Here's the drawing with two shaded views (mm, measured from the low corner). I have some questions. A direction names the side the tool comes from. Round coordinates to 2 decimals unless told otherwise and drop trailing zeros. Write each loop counter-clockwise with the first axis right and the second up, starting at its lowest first coordinate (ties: lowest second). Pieces come first, ordered by that corner, then holes.
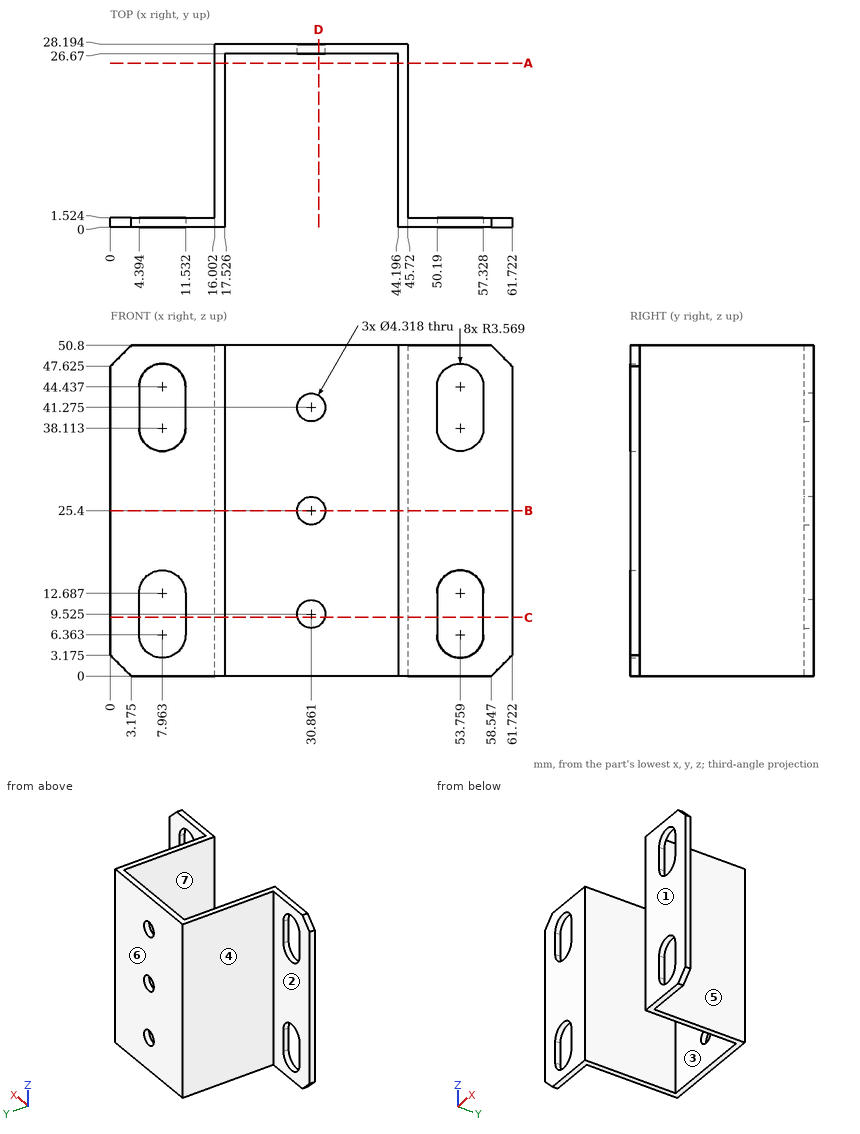
Q1. We'd pull the mould along X, two halves only. Please class the marked faces 4, 5, 6 and 7: pulls with the +X half, pulls with the -X half, needs draft (parallel to the pull), parting line crosses it, or undercut.
Q2. Imagine slicing it at A-A, the plane y = 25.25. Write out the boundary of the cut face in (x, z), then the cut area to 3 significant figures.
Q3. I'm going to push flat-ended pins straight in: pin 1 Ø8 at (y, z) = (23.5, 18.5) entering from +X; pin 2 Ø5 at (x, y) = (12.5, 24.5) entering from -Z; pin 3 Ø13 at (x, z) = (53.5, 37.5) entering from +Y; pin 4 Ø1.7 at (y, z) = (1, 9) entering from -X. Where does each tip first touch, or does it pass through?
Q4. On a 3-axis mill with a long thin cutter (end or side, diameter ignored), from which of +Z, -Z, +X, -X, +Y, -Y can I reach the whole of each face in a straight line? I mean the marked faces 1, 2 and 3. Say none if no direction works.
Q5. Imagine slicing it at C-C, the plane z = 9. Write out the boundary of the cut face in (x, y) (1 decimal).
Q6. If I drill on L1, parallel to X at y = 16.25, z = 28; L2, parallel to X at y = 27.15, z = 25.4; L3, parallel to Y at x = 34, z = 23, over which ranges is the centre line in solid material (lowest first)?
Q7. Imagine slicing it at D-D, the plane x = 32. Write out the boundary of the cut face in (y, z).
Q8. Imagine slicing it at B-B, the plane z = 25.4. Write out the boundary of the cut face in (x, y), then the cut area to 3 significant figures.
Results found:
1. face 4: pulls with the -X half
1. face 5: pulls with the +X half
1. face 6: needs draft
1. face 7: undercut
2. outline: (16, 0) - (17.53, 0) - (17.53, 50.8) - (16, 50.8) - close; (44.2, 0) - (45.72, 0) - (45.72, 50.8) - (44.2, 50.8) - close
2. area: 155 mm2
3. pin 1: stops at x = 45.72
3. pin 2: passes through
3. pin 3: stops at y = 1.52
3. pin 4: stops at x = 0
4. face 1: +Z, -Z, +X, -X, -Y
4. face 2: +Z, -Z, -X, +Y
4. face 3: +Z, -Z, -Y
5. outline: (0, 0) - (4.4, 0) - (4.4, 1.5) - (0, 1.5) - close; (11.5, 0) - (17.5, 0) - (17.5, 26.7) - (28.8, 26.7) - (28.8, 28.2) - (16, 28.2) - (16, 1.5) - (11.5, 1.5) - close; (33, 26.7) - (44.2, 26.7) - (44.2, 0) - (50.2, 0) - (50.2, 1.5) - (45.7, 1.5) - (45.7, 28.2) - (33, 28.2) - close; (57.3, 0) - (61.7, 0) - (61.7, 1.5) - (57.3, 1.5) - close
6. L1: x = 16 to 17.53, 44.2 to 45.72
6. L2: x = 16 to 28.7, 33.02 to 45.72
6. L3: y = 26.67 to 28.19
7. outline: (26.67, 0) - (28.19, 0) - (28.19, 7.69) - (26.67, 7.69) - close; (26.67, 11.36) - (28.19, 11.36) - (28.19, 23.57) - (26.67, 23.57) - close; (26.67, 27.23) - (28.19, 27.23) - (28.19, 39.44) - (26.67, 39.44) - close; (26.67, 43.11) - (28.19, 43.11) - (28.19, 50.8) - (26.67, 50.8) - close
8. outline: (0, 0) - (17.53, 0) - (17.53, 26.67) - (28.7, 26.67) - (28.7, 28.19) - (16, 28.19) - (16, 1.52) - (0, 1.52) - close; (33.02, 26.67) - (44.2, 26.67) - (44.2, 0) - (61.72, 0) - (61.72, 1.52) - (45.72, 1.52) - (45.72, 28.19) - (33.02, 28.19) - close
8. area: 169 mm2
